from build123d import *

# Parameters (mm, degrees)
SKETCH2_W                = 13
SKETCH2_H                = 16
SKETCH2_R                = 2
BOSS_EXTRUDE1_DEPTH      = 6
BOSS_EXTRUDE2_DEPTH      = 3
BOSS_EXTRUDE2_DEPTH_BACK = 3
SKETCH6_R                = 5
BOSS_EXTRUDE4_DEPTH      = 15
BOSS_EXTRUDE4_DEPTH_BACK = 15
SKETCH7_R                = 2.5
CUT_EXTRUDE2_DEPTH       = 31
FILLET3_R                = 0.5
FILLET4_R                = 0.5
SKETCH10_R               = 1.5
CUT_EXTRUDE3_DEPTH       = 4


with BuildPart() as part:
    # Sketch2 → Boss-Extrude1 (new body)
    with BuildSketch(Plane.XY):
        with Locations((-6.5, 8)):
            Rectangle(SKETCH2_W, SKETCH2_H)
        with Locations((-8, 8)):
            Circle(SKETCH2_R, mode=Mode.SUBTRACT)
        with Locations((6.5, 8)):
            Rectangle(SKETCH2_W, SKETCH2_H)
        with Locations((8, 8)):
            Circle(SKETCH2_R, mode=Mode.SUBTRACT)
    extrude(amount=BOSS_EXTRUDE1_DEPTH)

    # Sketch3 → Boss-Extrude2 (add, two sides)
    with BuildSketch(Plane(origin=(0, 0, 0), x_dir=(0, 0, -1), z_dir=(1, 0, 0))) as boss_extrude2_sk:
        with BuildLine():
            Line((-6, 0), (-8, 0))
            ThreePointArc((-8, 0), (-14.363961031, 2.636038969), (-17, 9))
            Line((-17, 9), (-17, 44))
            Line((-17, 44), (-6, 44))
            Line((-6, 44), (-6, 16))
            Line((-6, 16), (-6, 0))
        make_face()
    extrude(amount=BOSS_EXTRUDE2_DEPTH)
    extrude(boss_extrude2_sk.sketch, amount=-BOSS_EXTRUDE2_DEPTH_BACK)

    # Sketch6 → Boss-Extrude4 (add, two sides)
    with BuildSketch(Plane(origin=(0, 0, 6), x_dir=(-1, 0, 0), z_dir=(0, 0, -1))) as boss_extrude4_sk:
        with Locations((0, 44)):
            Circle(SKETCH6_R)
    extrude(amount=BOSS_EXTRUDE4_DEPTH)
    extrude(boss_extrude4_sk.sketch, amount=-BOSS_EXTRUDE4_DEPTH_BACK)

    # Sketch7 → Cut-Extrude2 (cut, through all)
    with BuildSketch(Plane(origin=(0, 0, -9), x_dir=(-1, 0, 0), z_dir=(0, 0, -1))):
        with Locations((0, 44)):
            Circle(SKETCH7_R)
    extrude(amount=-CUT_EXTRUDE2_DEPTH, mode=Mode.SUBTRACT)

    # Fillet3
    fillet3_edges = [part.edges().sort_by_distance(p)[0] for p in [
        (5, 44, 21),
        (5, 44, -9),
    ]]
    fillet(fillet3_edges, radius=FILLET3_R)

    # Fillet4
    fillet4_edges = [part.edges().sort_by_distance(p)[0] for p in [
        (3, 40, 11.5),
        (-3, 40, 11.5),
    ]]
    fillet(fillet4_edges, radius=FILLET4_R)

    # Sketch10 → Cut-Extrude3 (cut)
    with BuildSketch(Plane.ZX.offset(49)):
        with Locations((6.569879023, 0)):
            Circle(SKETCH10_R)
    extrude(amount=-CUT_EXTRUDE3_DEPTH, mode=Mode.SUBTRACT)


solid = part.part
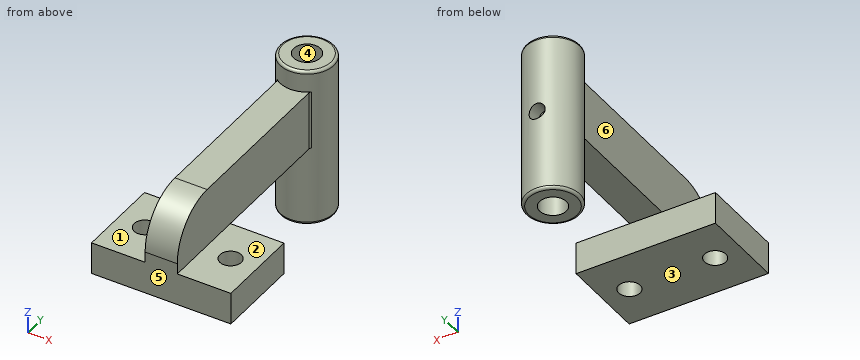
Could you check a few things on this model? Use its own coordinates, in mm. Face numbers are marked on the shaded views. A direction names the side the tool comes from. Coordinates: 2 decimals unless noted, no trailing zeros. Order: outer loops, then holes, each group sorted by start corner. A loop starts at its lowest first (then second) coordinate and runs counter-clockwise, first axis right, second up.
Q1. Which directions (+Z, -Z, +X, -X, +Y, -Y) give clear straight access to the entire face, cutting with the end or side of a thin tool? Please do the marked faces 1, 2 and 3.
Q2. Suppose I cut it at A-A on z = 3. Please give me the cut outline in (x, y).
Q3. Will these pins go through, and if not, where does the flat tip stop? pin 1 (4 mm diameter, centred on y = 40.5, z = 18, fed in from -X); pin 2 (8 mm diameter, centred on x = 0, y = 44, fed in from +Z); pin 3 (1.5 mm diameter, centred on y = 18, z = 9.5, fed in from +X); pin 4 (12 mm diameter, centred on y = 20.5, z = 12, fed in from -X).
Q4. Suppose I cut it at C-C on z = -5. Please give me the cut outline in (x, y), and give its area (3 significant figures).
Q5. Suppose I cut it at B-B on x = -8. Please give me the cut outline in (y, z).
Q6. Thinking about a two-plate mould opening in X: for the marked faces 4, 5 and 6, which applies, released by +X, released by -X, zero draft, split by the parting line, or undercut?
Q7. Suppose I cut it at D-D on y = 3. Please give me the cut outline in (x, z).
Q8. Please list where these lines run through material, in increasing order: L1, parallel to Y at x = 0, z = 1.5; L2, parallel to Y at x = 8, z = 2.35; L3, parallel to Y at x = -1.5, z = 5.
Answer:
1. face 1: +Z, -X, -Y
1. face 2: +Z, +X, -Y
1. face 3: -Z, +X, -X, -Y
2. outline: (-13, 0) - (13, 0) - (13, 16) - (-13, 16) - close; circle Ø10 at (0, 44); hole circle Ø4 at (-8, 8); hole circle Ø5 at (0, 44); hole circle Ø4 at (8, 8)
3. pin 1: stops at x = -4.77
3. pin 2: stops at z = 21
3. pin 3: stops at x = 3
3. pin 4: stops at x = -3
4. outline: circle Ø10 at (0, 44); hole circle Ø5 at (0, 44)
4. area: 58.9 mm2
5. outline: (0, 0) - (6, 0) - (6, 6) - (0, 6) - close; (10, 0) - (16, 0) - (16, 6) - (10, 6) - close
6. face 4: undercut
6. face 5: zero draft
6. face 6: released by -X
7. outline: (-13, 0) - (13, 0) - (13, 6) - (3, 6) - (3, 14.71) - (-3, 14.71) - (-3, 6) - (-13, 6) - close
8. L1: y = 0 to 16, 39 to 41.5, 46.5 to 49
8. L2: y = 0 to 6, 10 to 16
8. L3: y = 0 to 16, 39.23 to 42, 46 to 48.77
